Part model, mm, in its own coordinate system. A direction names the side the tool comes from. Round coordinates to 2 decimals unless told otherwise and drop trailing zeros. Loops run counter-clockwise (first coordinate to the right, second up) from the corner with the lowest first, then second, coordinate; pieces in that order, holes last.
(1) Cut at A-A on x = 0. List the corners of the cut face in (y, z) (3 decimals).
(2) Cut at B-B on y = 0. List the corners of the cut face in (x, z) (3 decimals).
(3) Mould opens along X. For faces 1 (the face through (22.537, 22.505, -35.164)), 2 (the face through (7.33, -14.08, -34.44)), 3 (the face through (-1, -22, -69.85)), 4 (the face through (0, -13, 0)) say: +X half, -X half, draft (parallel to the pull), parting line (faces both ways), or undercut.
(4) Probe probe 1 along X at (y, z) = (0, -22) (3 decimals); probe 2 along Z at (x, y) = (16.5, 2); probe 3 along Y at (x, z) = (19, -26). List the from-to ranges inside material, lowest first.
(5) Cut at C-C on z = -45.5. List the corners of the cut face in (x, y) (3 decimals).
(6) Tool access for faces 5 (the face through (16.788, 19.033, -47.592)), 6 (the face through (19.033, 16.788, -47.592)), 7 (the face through (-19.033, -16.788, -47.592)), 8 (the face through (-16.788, -19.033, -47.592)): list every direction of +Z, -Z, +X, -X, +Y, -Y with a clear straight run to the whole face (end or side of a thin tool).
(7) Flat gauge pins, fed straight in: pin 1 (1.3 mm diameter, centred on x = -0.5, y = 13, fed in from +Z); pin 2 (10 mm diameter, centred on y = 11, z = -32, fed in from +X); pin 3 (5.5 mm diameter, centred on x = 0, y = 34.35, fed in from +Z); pin 4 (6 mm diameter, centred on y = -10.5, z = -20, fed in from -X). Where does each tip first touch, or does it go through?
(8) Cut at D-D on z = -60.5. List the corners of the cut face in (x, y) (3 decimals), then the cut area to 3 significant figures.
from build123d import *

# Parameters (mm, degrees)
SKETCH1_R         = 15.875
SKETCH1_R_2       = 12.7
EXTRUDE1_DEPTH    = 76.2
EXTRUDE2_DEPTH    = 25.4
EXTRUDE3_START    = 6.35
SKETCH3_R         = 50.8
SKETCH3_R_2       = 15.875
EXTRUDE3_DEPTH    = 6.35
SKETCH4_R         = 3.175
EXTRUDE5_DEPTH    = 7.62
RIB4_REACH        = 106.727
SKETCH6_WALL_W    = 287.037040946
SKETCH6_WALL_H    = 3.175
CIRPATTERN1_COUNT = 4


with BuildPart() as part:
    # Sketch1 → Extrude1 (new body)
    with BuildSketch(Plane.XY):
        Circle(SKETCH1_R)
        Circle(SKETCH1_R_2, mode=Mode.SUBTRACT)
    extrude(amount=-EXTRUDE1_DEPTH)

    # Sketch2 → Extrude2 (cut)
    with BuildSketch(Plane.XY):
        Polygon((1.778, 12.7), (1.778, 14.224), (-1.778, 14.224), (-1.778, 12.7), (-1.778, 12.361177694), (1.778, 12.361177694), align=None)
    extrude(amount=-EXTRUDE2_DEPTH, mode=Mode.SUBTRACT)

    # Sketch3 → Extrude3 (add)
    with BuildSketch(Plane.XY.offset(-76.2).offset(EXTRUDE3_START)):
        Circle(SKETCH3_R)
        Circle(SKETCH3_R_2, mode=Mode.SUBTRACT)
    extrude(amount=-EXTRUDE3_DEPTH)

    # Sketch4 → Extrude5 (cut)
    with BuildSketch(Plane.XY.offset(-76.2)):
        with Locations(Location((0, 34.350268622, 0), (0, 0, 180))):
            Circle(SKETCH4_R)
        with Locations(Location((34.350268622, 0, 0), (0, 0, 180))):
            Circle(SKETCH4_R)
        with Locations(Location((0, -34.350268622, 0), (0, 0, 180))):
            Circle(SKETCH4_R)
        with Locations(Location((-34.350268622, 0, 0), (0, 0, 180))):
            Circle(SKETCH4_R)
    extrude(amount=EXTRUDE5_DEPTH, mode=Mode.SUBTRACT)

    # Sketch6 wall → Rib4 (add, up to next)
    with BuildSketch(Plane(origin=(22.710403549, -22.710403549, -35.726788107), x_dir=(0.303905417501, -0.303905417501, -0.902930226777), z_dir=(-0.638468086292, 0.638468086292, -0.429787163108)), mode=Mode.PRIVATE) as rib4_sk1:
        Rectangle(SKETCH6_WALL_W, SKETCH6_WALL_H)
    rib4_tool1 = extrude(rib4_sk1.sketch, amount=RIB4_REACH, mode=Mode.PRIVATE) - part.part
    rib4 = rib4_tool1.solids().sort_by_distance((22.710403549, -22.710403549, -35.726788107))[0]
    add(rib4)

    # CirPattern1: Rib4 ×4 about axis
    cirpattern1_axis = Axis((0, 0, 0), (0, 0, 1))
    for i in range(1, CIRPATTERN1_COUNT):
        add(rib4.rotate(cirpattern1_axis, i * 360 / CIRPATTERN1_COUNT))


solid = part.part
Final values:
1. outline: (-50.8, -76.2) - (-37.525, -76.2) - (-37.525, -69.85) - (-50.8, -69.85) - close; (-31.175, -76.2) - (-12.7, -76.2) - (-12.7, 0) - (-15.875, 0) - (-15.875, -69.85) - (-31.175, -69.85) - close; (12.7, -76.2) - (31.175, -76.2) - (31.175, -69.85) - (15.875, -69.85) - (15.875, 0) - (14.224, 0) - (14.224, -25.4) - (12.7, -25.4) - close; (37.525, -76.2) - (50.8, -76.2) - (50.8, -69.85) - (37.525, -69.85) - close
2. outline: (-50.8, -76.2) - (-37.525, -76.2) - (-37.525, -69.85) - (-50.8, -69.85) - close; (-31.175, -76.2) - (-12.7, -76.2) - (-12.7, 0) - (-15.875, 0) - (-15.875, -69.85) - (-31.175, -69.85) - close; (12.7, -76.2) - (31.175, -76.2) - (31.175, -69.85) - (15.875, -69.85) - (15.875, 0) - (12.7, 0) - close; (37.525, -76.2) - (50.8, -76.2) - (50.8, -69.85) - (37.525, -69.85) - close
3. face 1: +X half
3. face 2: undercut
3. face 3: undercut
3. face 4: draft
4. probe 1: x = -15.875 to -12.7, 12.7 to 15.875
4. probe 2: z = -76.2 to -69.85
4. probe 3: y = -19.87 to -16.75, 16.75 to 19.87
5. outline: (-27.122, -24.877) - (-24.877, -27.122) - (-10.047, -12.292) arc R15.875 ccw to (10.047, -12.292) - (24.877, -27.122) - (27.122, -24.877) - (12.292, -10.047) arc R15.875 ccw to (12.292, 10.047) - (27.122, 24.877) - (24.877, 27.122) - (10.047, 12.292) arc R15.875 ccw to (-10.047, 12.292) - (-24.877, 27.122) - (-27.122, 24.877) - (-12.292, 10.047) arc R15.875 ccw to (-12.292, -10.047) - close; hole circle Ø25.4 at (0, 0)
6. face 5: +Z, +Y
6. face 6: +Z, +X
6. face 7: +Z, -X
6. face 8: +Z, -Y
7. pin 1: stops at z = -25.4
7. pin 2: stops at x = 18.25
7. pin 3: passes through
7. pin 4: stops at x = -15.75
8. outline: (-32.171, -29.926) - (-29.926, -32.171) - (-10.047, -12.292) arc R15.875 ccw to (10.047, -12.292) - (29.926, -32.171) - (32.171, -29.926) - (12.292, -10.047) arc R15.875 ccw to (12.292, 10.047) - (32.171, 29.926) - (29.926, 32.171) - (10.047, 12.292) arc R15.875 ccw to (-10.047, 12.292) - (-29.926, 32.171) - (-32.171, 29.926) - (-12.292, 10.047) arc R15.875 ccw to (-12.292, -10.047) - close; hole circle Ø25.4 at (0, 0)
8. area: 641 mm2
